```python
from build123d import *

# Parameters (mm, degrees)
SKETCH_W      = 45
SKETCH_H      = 45
SKETCH_R      = 1.3
PAD_DEPTH     = 2
PAD001_DEPTH  = 45
SKETCH002_R   = 11.872
SKETCH002_R_2 = 1.6
POCKET_DEPTH  = 3.561
FILLET_R      = 5


with BuildPart() as part:
    # Sketch → Pad (new body)
    with BuildSketch(Plane.XY):
        Rectangle(SKETCH_W, SKETCH_H)
        with Locations((-18.15, 18.15)):
            Circle(SKETCH_R, mode=Mode.SUBTRACT)
        with Locations((-18.15, -18.15)):
            Circle(SKETCH_R, mode=Mode.SUBTRACT)
        with Locations((18.15, -18.15)):
            Circle(SKETCH_R, mode=Mode.SUBTRACT)
        with Locations((18.15, 18.15)):
            Circle(SKETCH_R, mode=Mode.SUBTRACT)
    extrude(amount=PAD_DEPTH)

    # Sketch001 (on Face3 of Pad) → Pad001 (join)
    with BuildSketch(Plane.XZ.offset(22.5)):
        Polygon((0, 0), (-4.74, 0), (-2.94, -1.56), (0, -1.56), (2.94, -1.56), (4.74, 0), align=None)
    extrude(amount=-PAD001_DEPTH)

    # Sketch002 (on Face13 of Pad001) → Pocket (cut, through all)
    with BuildSketch(Plane(origin=(0, 0, -1.56), x_dir=(1, 0, 0), z_dir=(0, 0, -1))):
        Circle(SKETCH002_R)
        with Locations((0, 17.186)):
            Circle(SKETCH002_R_2)
        with Locations((0, -17.186)):
            Circle(SKETCH002_R_2)
    extrude(amount=-POCKET_DEPTH, mode=Mode.SUBTRACT)

    # Fillet
    fillet_edges = [part.edges().sort_by_distance(p)[0] for p in [
        (22.5, -22.5, 1),
        (22.5, 22.5, 1),
        (-22.5, -22.5, 1),
        (-22.5, 22.5, 1),
    ]]
    fillet(fillet_edges, radius=FILLET_R)


solid = part.part
```
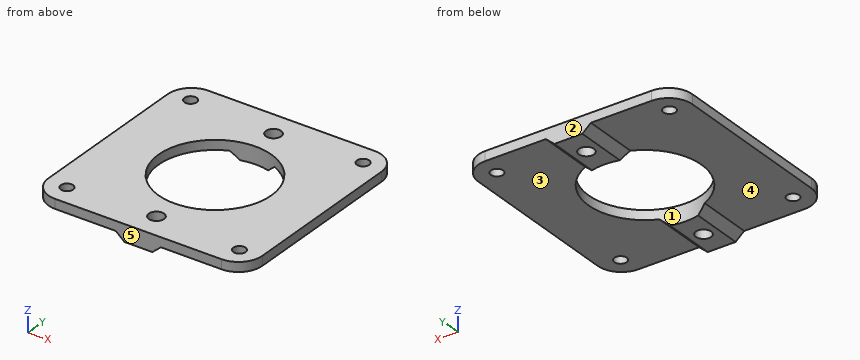
Here's how the part is built. I have some questions about the finished solid (model axes, mm). Face numbers are marked on the shaded views. A direction names the side the tool comes from. Round coordinates to 2 decimals unless told otherwise and drop trailing zeros. Write each loop counter-clockwise with the first axis right and the second up, starting at its lowest first coordinate (ties: lowest second). Pieces come first, ordered by that corner, then holes.
Q1. If we section it at A-A on x = 0: Write out the boundary of the cut face in (y, z), plus the area to 3 significant figures.
Q2. If we mould it in two halves opening along X, with no side actions, what happens to the marked faces 1 and 2? For each: +X half, -X half, draft (parallel to the pull), parting line (faces both ways), or undercut.
Q3. Which directions (+Z, -Z, +X, -X, +Y, -Y) give clear straight access to the entire face, cutting with the end or side of a thin tool? Please do the marked faces 3, 4 and 5.
Q4. If we section it at B-B on y = -9.5: Write out the boundary of the cut face in (x, z).
Q5. Please list where these lines run through material, in increasing order: probe 1 along Y at (x, z) = (0, 0.7); probe 2 along Y at (x, z) = (18.15, 0.7); probe 3 along X at (y, z) = (-0.5, 0.3).
Q6. Will these pins go through, and if not, where does the flat tip stop? P1, Ø2.5, axis at x = 0, y = 17.186, coming from the -Z side; P2, Ø14, axis at x = -11.5, y = 10.5, coming from the -Z side; P3, Ø10, axis at x = -18, y = 12, coming from the -Z side.
Q7. If we section it at C-C on y = 18.15: Write out the boundary of the cut face in (x, z), plus the area to 3 significant figures.
Q8. If we section it at D-D on z = -1.05: Write out the boundary of the cut face in (x, y), plus the area to 3 significant figures.
Answer below:
1. outline: (-22.5, -1.56) - (-18.79, -1.56) - (-18.79, 2) - (-22.5, 2) - close; (-15.59, -1.56) - (-11.87, -1.56) - (-11.87, 2) - (-15.59, 2) - close; (11.87, -1.56) - (15.59, -1.56) - (15.59, 2) - (11.87, 2) - close; (18.79, -1.56) - (22.5, -1.56) - (22.5, 2) - (18.79, 2) - close
1. area: 52.9 mm2
2. face 1: undercut
2. face 2: draft
3. face 3: -Z, +X, +Y, -Y
3. face 4: -Z, -X, +Y, -Y
3. face 5: +Z, -Z, +X, -X, -Y
4. outline: (-22.5, 0) - (-7.12, 0) - (-7.12, 2) - (-22.5, 2) - close; (7.12, 0) - (22.5, 0) - (22.5, 2) - (7.12, 2) - close
5. probe 1: y = -22.5 to -18.79, -15.59 to -11.87, 11.87 to 15.59, 18.79 to 22.5
5. probe 2: y = -22.46 to -19.45, -16.85 to 16.85, 19.45 to 22.46
5. probe 3: x = -22.5 to -11.86, 11.86 to 22.5
6. P1: passes through
6. P2: stops at z = -0.19
6. P3: stops at z = 0
7. outline: (-22.46, 0) - (-19.45, 0) - (-19.45, 2) - (-22.46, 2) - close; (-16.85, 0) - (-4.74, 0) - (-2.94, -1.56) - (-1.28, -1.56) - (-1.28, 2) - (-16.85, 2) - close; (1.28, -1.56) - (2.94, -1.56) - (4.74, 0) - (16.85, 0) - (16.85, 2) - (1.28, 2) - close; (19.45, 0) - (22.46, 0) - (22.46, 2) - (19.45, 2) - close
7. area: 82.3 mm2
8. outline: (-3.53, -22.5) - (3.53, -22.5) - (3.53, -11.34) arc R11.87 cw to (-3.53, -11.34) - close; (-3.53, 11.34) arc R11.87 cw to (3.53, 11.34) - (3.53, 22.5) - (-3.53, 22.5) - close; hole circle Ø3.2 at (0, -17.19); hole circle Ø3.2 at (0, 17.19)
8. area: 136 mm2
